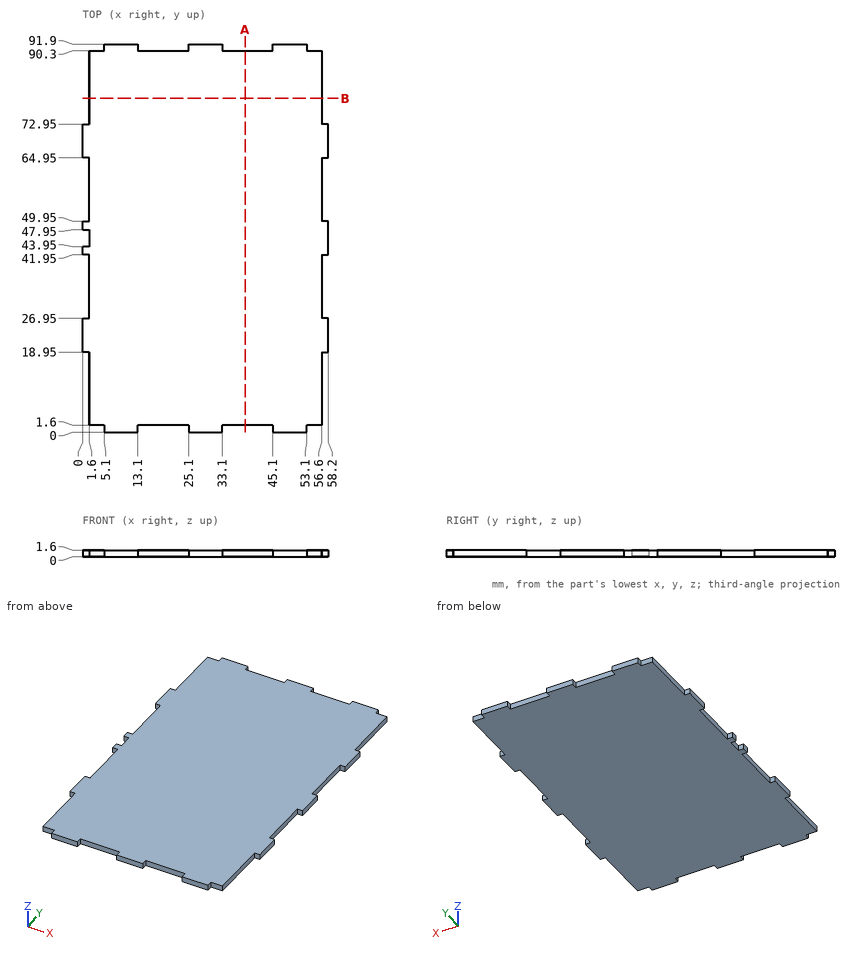
Check sheet for the drawn part. Datum: minimum x, y, z corner. Units: mm. Coordinates: 2 decimals unless noted, no trailing zeros. Write each loop counter-clockwise with the first axis right and the second up, starting at its lowest first coordinate (ties: lowest second). Pieces come first, ordered by that corner, then holes. Notation, with made-up numbers: (16, -1) - (43, -1) arc R27 ccw to (43, 34) - close; hole circle Ø7 at (-30, -20.75). An arc over 180 degrees is marked (long way). Answer as a JSON object with one key per item and string values.
(1) Cross-section at A-A on x = 38.5. Record the cut outline in (y, z).
Report:
{"outline": "(1.6, 0) - (90.3, 0) - (90.3, 1.6) - (1.6, 1.6) - close"}
(2) Gauge pin test, flat ends, axial feed: pin 1 Ø0.8 at (y, z) = (91.5, 0.5) entering from +X; pin 2 Ø0.5 at (y, z) = (91, 0.5) entering from -X; pin 3 Ø0.5 at (x, z) = (54.5, 1) entering from +Y. Record the tip position at first contact, or that the pin passes through.
Report:
{"pin 1": "x = 53.1", "pin 2": "x = 5.1", "pin 3": "y = 90.3"}
(3) Cross-section at B-B on y = 79. Record the cut outline in (x, z).
Report:
{"outline": "(1.6, 0) - (56.6, 0) - (56.6, 1.6) - (1.6, 1.6) - close"}
(4) Thickness scan on line 1 along X through (y, z) = (32.5, 0.5); line 2 along Y through (x, z) = (5, 0.45); line 3 along X through (y, z) = (45, 0.85). Record the ranges inside material, lowest first.
Report:
{"line 1": "1.6 to 56.6", "line 2": "1.6 to 90.3", "line 3": "1.6 to 58.2"}
